Source: CAD feature listing. Evaluate the final solid. Frame: model axes, mm. Face numbers are marked on the shaded views. A direction names the side the tool comes from. Round coordinates to 2 decimals unless told otherwise and drop trailing zeros. Order: outer loops, then holes, each group sorted by start corner. A loop starts at its lowest first (then second) coordinate and runs counter-clockwise, first axis right, second up. Notation, with made-up numbers: (76.5, 16) -> (133.5, 16) arc R22 cw to (133.5, 48) -> close; hole circle Ø10 at (59.5, -6.5). An arc over 180 degrees is marked (long way). Write item = value, one per line. Start each with the question number.
(1) Reachability of the marked faces 1 and 2 from +Z, -Z, +X, -X, +Y, -Y: full face, straight path, thin tool, end or side. Return the list, or none.
(2) Cut plane A-A on y = -5. Return the cut outline in (x, z).
(3) Contact query for flat-ended pins moving along their axis: pin 1 Ø0.5 at (y, z) = (1, 0) entering from -X; pin 2 Ø0.5 at (y, z) = (1, 0) entering from +X. Output: stop coordinate, or through.
(4) Ray query, line 1 (X direction, y = 1, z = -0.4); line 2 (Y direction, x = -0.6, z = -0.3); line 3 (Z direction, x = -1.5, y = 0.5). Return the intervals inside material, ascending.
(5) Draft query along Z for the marked faces 3, 4 and 5. Return one class per face: released by +Z, released by -Z, zero draft, split by the parting line, or undercut.
from build123d import *

# Parameters (mm, degrees)
SKETCH_1_R          = 2.85
EXTRUDE_1_DEPTH     = 1.6
CUT_EXTRUDE_1_DEPTH = 1
FILLET_1_R          = 1.5
SKETCH_3_R          = 1.4
EXTRUDE_2_DEPTH     = 6
CHAMFER_1_SIZE      = 0.2


with BuildPart() as part:
    # 草图1 → 凸台-拉伸1 (new body)
    with BuildSketch(Plane(origin=(0, 0, 0), x_dir=(1, 0, 0), z_dir=(0, 1, 0))):
        Circle(SKETCH_1_R)
    extrude(amount=EXTRUDE_1_DEPTH)

    # 草图2 → 切除-拉伸1 (cut)
    with BuildSketch(Plane(origin=(0, 1.6, 0), x_dir=(1, 0, 0), z_dir=(0, 1, 0))):
        Polygon((0, -1.154700538), (1, -0.577350269), (1, 0.577350269), (0, 1.154700538), (-1, 0.577350269), (-1, -0.577350269), align=None)
    extrude(amount=-CUT_EXTRUDE_1_DEPTH, mode=Mode.SUBTRACT)

    # 圆角1
    fillet_1_edges = [part.edges().sort_by_distance(p)[0] for p in [
        (-2.85, 1.6, 0),
    ]]
    fillet(fillet_1_edges, radius=FILLET_1_R)

    # 草图3 → 凸台-拉伸2 (add)
    with BuildSketch(Plane.XZ):
        Circle(SKETCH_3_R)
    extrude(amount=EXTRUDE_2_DEPTH)

    # 倒角1
    chamfer_1_edges = [part.edges().sort_by_distance(p)[0] for p in [
        (-1.4, -6, 0),
    ]]
    chamfer(chamfer_1_edges, length=CHAMFER_1_SIZE)


solid = part.part
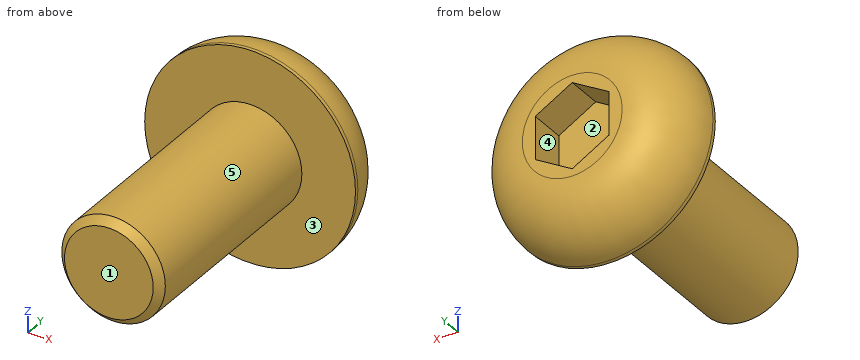
Evaluation:
q1.face_1 = +Z, -Z, +X, -X, -Y
q1.face_2 = +Y
q2.outline = circle Ø2.8 at (0, 0)
q3.pin_1 = -2.7
q3.pin_2 = 2.7
q4.line_1 = -2.52 to -1, 1 to 2.52
q4.line_2 = -6 to 0.6
q4.line_3 = -2.36 to 2.36
q5.face_3 = zero draft
q5.face_4 = undercut
q5.face_5 = split by the parting line
